Read the model definition and answer for the solid it produces. Units are mm, in the model's axes. Coordinates: 2 decimals unless noted, no trailing zeros. Use one line per item in the form item = value. Start each with the question number.
from build123d import *

# Parameters (mm, degrees)
SCHIZZO1_W                   = 184
SCHIZZO1_H                   = 200.217102587
ESTRUSIONE_ESTRUSIONE1_DEPTH = 4
M8_CLEARANCE_HOLE2_D         = 8.4


with BuildPart() as part:
    # Schizzo1 → Estrusione-Estrusione1 (new body)
    with BuildSketch(Plane.XY.offset(218.103339909)):
        with Locations((62.879048982, -170.411757868)):
            Rectangle(SCHIZZO1_W, SCHIZZO1_H)
    extrude(amount=ESTRUSIONE_ESTRUSIONE1_DEPTH)

    # M8 Clearance Hole2 (through all)
    with Locations(Plane(origin=(0, 0, 218.103339909), x_dir=(1, 0, 0), z_dir=(0, 0, -1))):
        with Locations((91.897840875, 70.752400597), (69.897840875, 70.752400597), (91.897840875, 108.752400597), (69.897840875, 108.752400597)):
            Hole(M8_CLEARANCE_HOLE2_D / 2)


solid = part.part
Q1. For a pull along Y with two mould halves and no side action, classify faces 1 (the flat face through (62, -169, 218.103)), 2 (the cylindrical face through (88.02, -107.14, 220.13)) as +Y half, -Y half, draft (parallel to the pull), parting line (faces both ways), or undercut.
Q2. Consider probe 1 along Y at (x, z) = (70.5, 218.4); probe 2 along Y at (x, z) = (73.5, 220.55). Determine where each line is inside the solid, lowest interval first.
Q3. Given P1, Ø13.5, axis at x = 91.9, y = -70.75, coming from the +Z side, flat-ended and moving along its own axis, determine where the tip first touches the part or whether it passes through.
Result sheet:
q1.face_1 = draft
q1.face_2 = undercut
q2.probe_1 = -270.52 to -112.91, -104.6 to -74.91
q2.probe_2 = -270.52 to -110.91, -106.59 to -72.91
q3.P1 = 222.1
